The listing builds one solid part. Answer for the finished solid, in the listing's coordinates (mm). Give positions to 0.01 mm unless a question says otherwise; leave off trailing zeros. Write each question's results on one line, items separated by ' | '.
from build123d import *

# Parameters (mm, degrees)
BOSS_EXTRUDE1_DEPTH = 3
SKETCH2_R           = 1.5
CUT_EXTRUDE1_DEPTH  = 115.861021763
SKETCH3_R           = 3
CUT_EXTRUDE2_DEPTH  = 2.3


with BuildPart() as part:
    # Sketch1 → Boss-Extrude1 (new body)
    with BuildSketch(Plane.XY):
        with BuildLine():
            Line((-98.454935622, 37.703862661), (1.545064378, 37.703862661))
            ThreePointArc((1.545064378, 37.703862661), (8.61613219, 34.774930473), (11.545064378, 27.703862661))
            Line((11.545064378, 27.703862661), (11.545064378, -22.296137339))
            ThreePointArc((11.545064378, -22.296137339), (8.61613219, -29.367205151), (1.545064378, -32.296137339))
            Line((1.545064378, -32.296137339), (-98.454935622, -32.296137339))
            ThreePointArc((-98.454935622, -32.296137339), (-105.526003434, -29.367205151), (-108.454935622, -22.296137339))
            Line((-108.454935622, -22.296137339), (-108.454935622, 27.703862661))
            ThreePointArc((-108.454935622, 27.703862661), (-105.526003434, 34.774930473), (-98.454935622, 37.703862661))
        make_face()
    extrude(amount=BOSS_EXTRUDE1_DEPTH)

    # Sketch2 → Cut-Extrude1 (cut, through all)
    with BuildSketch(Plane.XY.offset(3)):
        with Locations((-54.454935622, 31.60657407)):
            Circle(SKETCH2_R)
        with Locations((-42.454935622, 31.60657407)):
            Circle(SKETCH2_R)
        with Locations((-70.454935622, -15.296137339)):
            Circle(SKETCH2_R)
        with Locations((-70.454935622, -27.296137339)):
            Circle(SKETCH2_R)
        with Locations((-26.454935622, -15.296137339)):
            Circle(SKETCH2_R)
        with Locations((-26.454935622, -27.296137339)):
            Circle(SKETCH2_R)
    extrude(amount=-CUT_EXTRUDE1_DEPTH, mode=Mode.SUBTRACT)

    # Sketch3 → Cut-Extrude2 (cut)
    with BuildSketch(Plane.XY.offset(3)):
        with Locations((-102.954935622, 23.203862661)):
            Circle(SKETCH3_R)
        with Locations((-102.954935622, 3.203862661)):
            Circle(SKETCH3_R)
        with Locations((3.545064378, 24.203862661)):
            Circle(SKETCH3_R)
        with Locations((3.545064378, 2.203862661)):
            Circle(SKETCH3_R)
    extrude(amount=-CUT_EXTRUDE2_DEPTH, mode=Mode.SUBTRACT)


solid = part.part
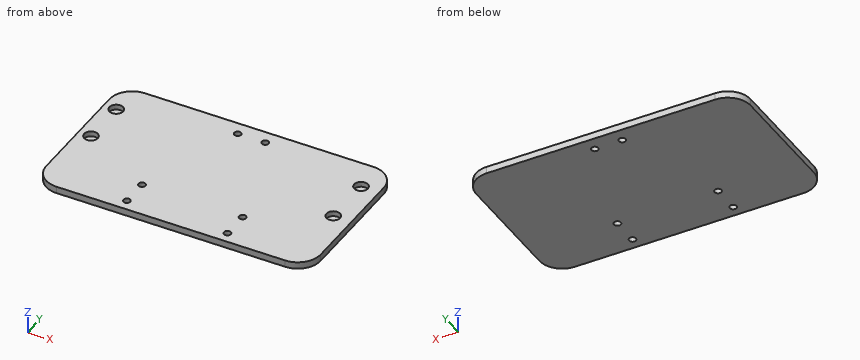
Item 1: Find the intervals of material crossed by line 1 along X through (y, z) = (3.5, 1.85); line 2 along X through (y, z) = (-15, 1.8); line 3 along Y through (x, z) = (-71.5, 0.25), in increasing order. Write a range as [from, to].
Values found:
line 1: x = [-108.45, -105.94], [-99.97, 0.84], [6.25, 11.55] | line 2: x = [-108.45, -71.93], [-68.98, -27.93], [-24.98, 11.55] | line 3: y = [-32.3, -28.37], [-26.22, -16.37], [-14.22, 37.7]
Item 2: A flat-ended cylindrical pin translates along its axis: P1, Ø1.8, axis at x = 2, y = 25, coming from the +Z side. Find the tip coordinate at first contact, or state that the pin passes through.
Values found:
P1: stops at z = 0.7
Item 3: A cutting plane is placed at A-A, the plane z = 1.25. Count the separate pieces of the cut face and the enclosed holes in it, plus the area to 3 significant figures.
Values found:
separate pieces: 1 | enclosed holes: 10 | area: 8,160 mm²
